Geometry check sheet. Reference: drawing and pictorial views, mm from the part's lowest x, y, z. Coordinates: 2 decimals unless noted, no trailing zeros. Write each loop counter-clockwise with the first axis right and the second up, starting at its lowest first coordinate (ties: lowest second). Pieces come first, ordered by that corner, then holes. Notation, with made-up numbers: (73.5, 16) -> (118.5, 16) arc R26 cw to (118.5, 37) -> close; hole circle Ø1 at (-4, 7.5). An arc over 180 degrees is marked (long way). Put each result on its own line as item: value.
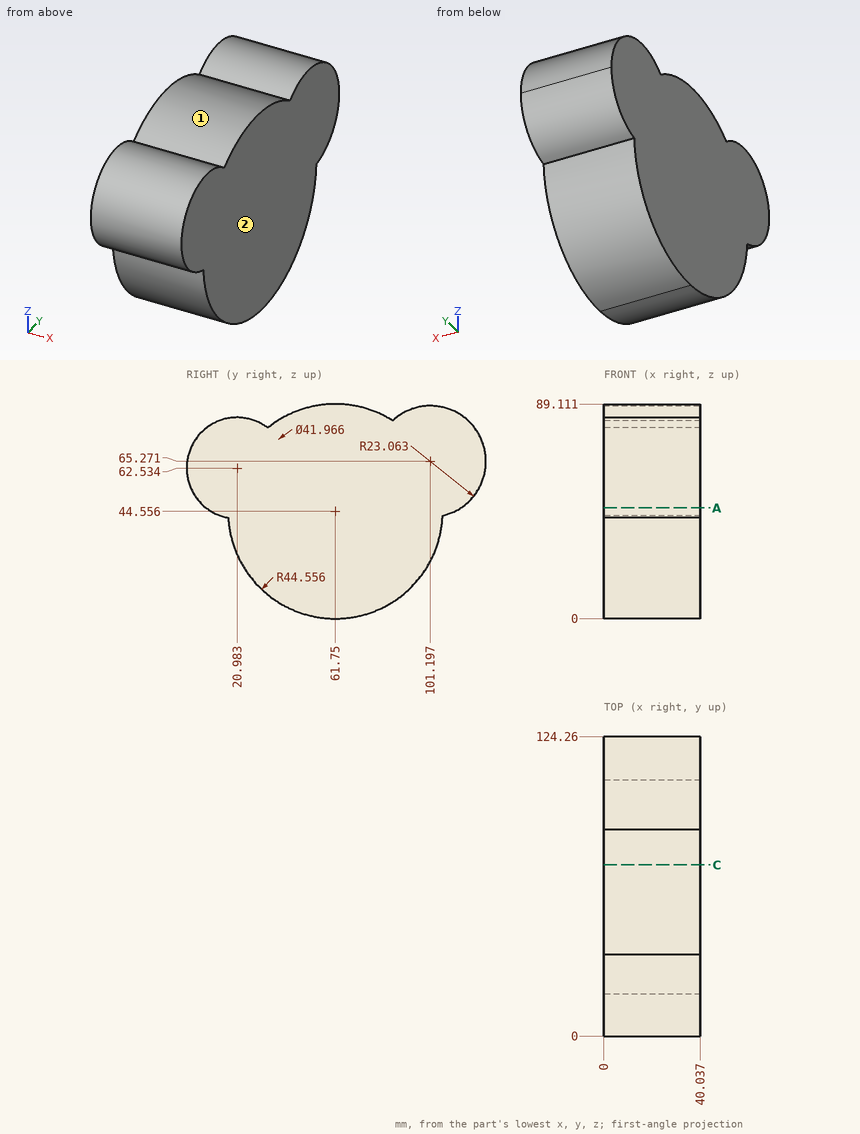
Q1. Cross-section at C-C (y = 71). Record the cut outline in (x, z), plus the area to 3 significant figures.
Recorded:
outline: (0, 0.97) -> (40.04, 0.97) -> (40.04, 88.14) -> (0, 88.14) -> close
area: 3,490 mm2
Q2. Material ranges on line 1 along Z through (x, y) = (7.5, 72.5) (1 decimal); line 2 along Z through (x, y) = (2.5, 23) (1 decimal); line 3 along Y through (x, z) = (12, 10.5), recorded low to high.
Recorded:
line 1: z = 1.3 to 87.8
line 2: z = 22.6 to 83.4
line 3: y = 33.02 to 90.48
Q3. Mould release check, pull along Y, two halves, no side actions. Record for the marked faces 1 and 2: released by +Y, released by -Y, zero draft, split by the parting line, or undercut.
Recorded:
face 1: undercut
face 2: zero draft
Q4. Cross-section at A-A (z = 46). Record the cut outline in (x, y).
Recorded:
outline: (0, 8.06) -> (40.04, 8.06) -> (40.04, 113.87) -> (0, 113.87) -> close
Q5. Depth check by flat-ended pin: P1, Ø6, axis at x = 26.5, y = 78, coming from the +Z side (1 decimal); P2, Ø8, axis at x = 26, z = 18, coming from the -Y side (1 decimal); P3, Ø4, axis at x = 22, y = 75.5, coming from the -Z side. Enter the tip coordinate at first touch or a pass-through.
Recorded:
P1: stops at z = 87.1
P2: stops at y = 23.3
P3: stops at z = 1.58
